Design review of the part shown in the three views and the two pictorial views. Dimensions are in mm from the part's minimum x, y and z. A direction names the side the tool comes from. Give positions to 0.01 mm unless a question says otherwise; leave off trailing zeros. Order: outer loops, then holes, each group sorted by start corner. A loop starts at its lowest first (then second) coordinate and runs counter-clockwise, first axis right, second up.
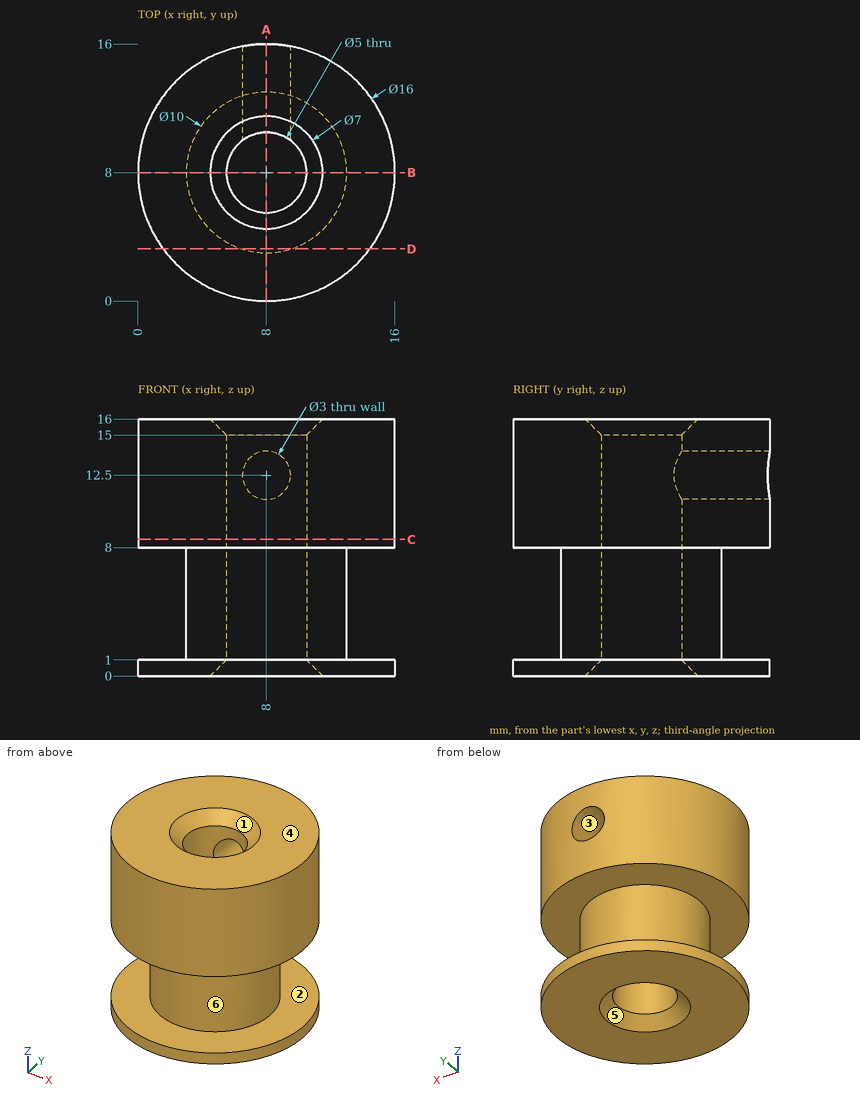
Item 1: Draft analysis for pull direction Y (two halves, no side actions). For the marked faces 4, 5 and 6, state which applies: released by +Y, released by -Y, zero draft, split by the parting line, or undercut.
Values found:
face 4: zero draft
face 5: undercut
face 6: split by the parting line
Item 2: For line 1 (Z direction, x = 8, y = 14.25); line 2 (Z direction, x = 14, y = 8.5); line 3 (Z direction, x = 8.5, y = 13.75), list the stretches that pass through material, from the lowest coordinate up.
Values found:
line 1: z = 0 to 1, 8 to 11, 14 to 16
line 2: z = 0 to 1, 8 to 16
line 3: z = 0 to 1, 8 to 11.09, 13.91 to 16
Item 3: Take a section at B-B (y = 8). Give the boundary of the cut face in (x, z).
Values found:
outline: (0, 0) - (4.5, 0) - (5.5, 1) - (5.5, 15) - (4.5, 16) - (0, 16) - (0, 8) - (3, 8) - (3, 1) - (0, 1) - close; (10.5, 1) - (11.5, 0) - (16, 0) - (16, 1) - (13, 1) - (13, 8) - (16, 8) - (16, 16) - (11.5, 16) - (10.5, 15) - close
Item 4: Take a section at C-C (z = 8.5). Give the boundary of the cut face in (x, y).
Values found:
outline: circle Ø16 at (8, 8); hole circle Ø5 at (8, 8)
Item 5: For the marked faces 1, 2 and 3, list the 3-axis set-ups (+Z, -Z, +X, -X, +Y, -Y) from which the entire face can be reached by the end or side of a thin tool; tool diameter is ignored.
Values found:
face 1: +Z
face 2: none
face 3: +Y
Item 6: Take a section at D-D (y = 3.25). Give the boundary of the cut face in (x, z).
Values found:
outline: (1.56, 0) - (14.44, 0) - (14.44, 1) - (9.56, 1) - (9.56, 8) - (14.44, 8) - (14.44, 16) - (1.56, 16) - (1.56, 8) - (6.44, 8) - (6.44, 1) - (1.56, 1) - close
Item 7: Clearance check with flat-ended pins moving along their axes: pin 1 Ø1.5 at (x, z) = (13, 14) entering from +Y; pin 2 Ø5 at (y, z) = (6.5, 13.5) entering from -X; pin 3 Ø6 at (x, y) = (8, 8) entering from -Z; pin 4 Ø1 at (x, y) = (6, 9.5) entering from +Z. State where each tip first meets the part, or that it passes through.
Values found:
pin 1: stops at y = 14.78
pin 2: stops at x = 0
pin 3: stops at z = 0.5
pin 4: stops at z = 15.5
Item 8: Take a section at A-A (x = 8). Give the boundary of the cut face in (y, z).
Values found:
outline: (0, 0) - (4.5, 0) - (5.5, 1) - (5.5, 15) - (4.5, 16) - (0, 16) - (0, 8) - (3, 8) - (3, 1) - (0, 1) - close; (10.5, 1) - (11.5, 0) - (16, 0) - (16, 1) - (13, 1) - (13, 8) - (16, 8) - (16, 11) - (10.5, 11) - close; (10.5, 14) - (16, 14) - (16, 16) - (11.5, 16) - (10.5, 15) - close
